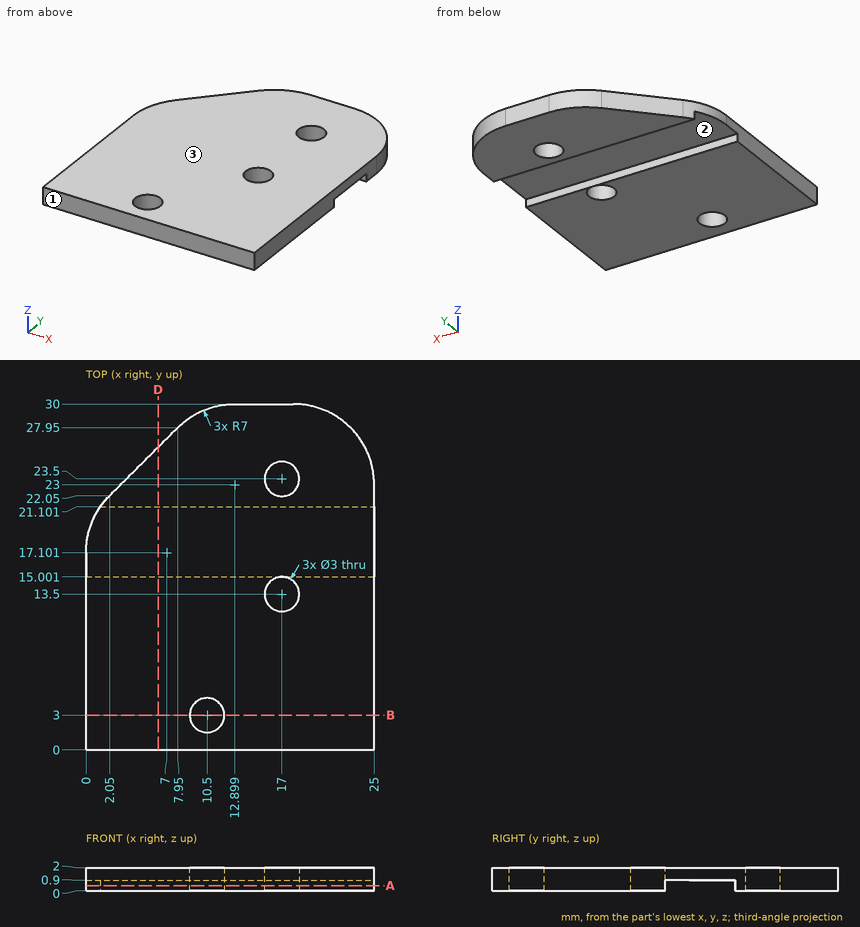
Study the drawing (mm; zero at the part's minimum x, y, z) and answer. Round coordinates to 2 decimals unless told otherwise and drop trailing zeros. Write each loop counter-clockwise with the first axis right and the second up, starting at its lowest first coordinate (ties: lowest second). Pieces come first, ordered by that corner, then holes. Notation, with made-up numbers: (26.25, -7.75) - (77.25, -7.75) arc R27 ccw to (77.25, 27.25) - close; hole circle Ø1 at (61.25, 17.25). An arc over 180 degrees is marked (long way). Use a Markdown table: item, result. Add a question column.
1. The part is cut by section A-A (z = 0.45). Give the number of separate pieces and of enclosed holes in the cut face, and give its area (3 significant figures).
2. Consider line 1 (Y direction, x = 10.5, z = 0.8) (1 decimal); line 2 (Y direction, x = 16.25, z = 0.2); line 3 (X direction, y = 3.5, z = 1.55) (1 decimal). Determine where each line is inside the solid, lowest interval first.
3. The part is cut by section B-B (y = 3). Write down the section's boundary in (x, z).
4. Flat-ended cylindrical pins translate along their axes: P1, Ø3, axis at x = 9, y = 18.5, coming from the -Z side; P2, Ø2.5, axis at x = 17, y = 13.5, coming from the +Z side. Find the tip coordinate at first contact, or state that the pin passes through.
5. For a pull along Y with two mould halves and no side action, classify the marked faces 1, 2 and 3 as +Y half, -Y half, draft (parallel to the pull), parting line (faces both ways), or undercut.
6. The part is cut by section D-D (x = 6.25). Write down the section's boundary in (y, z).
Reported:
| question | item | result |
|---|---|---|
| 1 | separate pieces | 2 |
| 1 | enclosed holes | 3 |
| 1 | area | 515 mm^2 |
| 2 | line 1 | 0 to 1.5, 4.5 to 15, 21.1 to 29.6 |
| 2 | line 2 | 0 to 12.2, 14.8 to 15, 21.1 to 22.2, 24.8 to 30 |
| 2 | line 3 | 0 to 9.1, 11.9 to 25 |
| 3 | outline | (0, 0) - (9, 0) - (9, 2) - (0, 2) - close; (12, 0) - (25, 0) - (25, 2) - (12, 2) - close |
| 4 | P1 | z = 0.9 |
| 4 | P2 | through |
| 5 | face 1 | -Y half |
| 5 | face 2 | undercut |
| 5 | face 3 | draft |
| 6 | outline | (0, 0) - (15, 0) - (15, 0.9) - (21.1, 0.9) - (21.1, 0) - (26.25, 0) - (26.25, 2) - (0, 2) - close |
